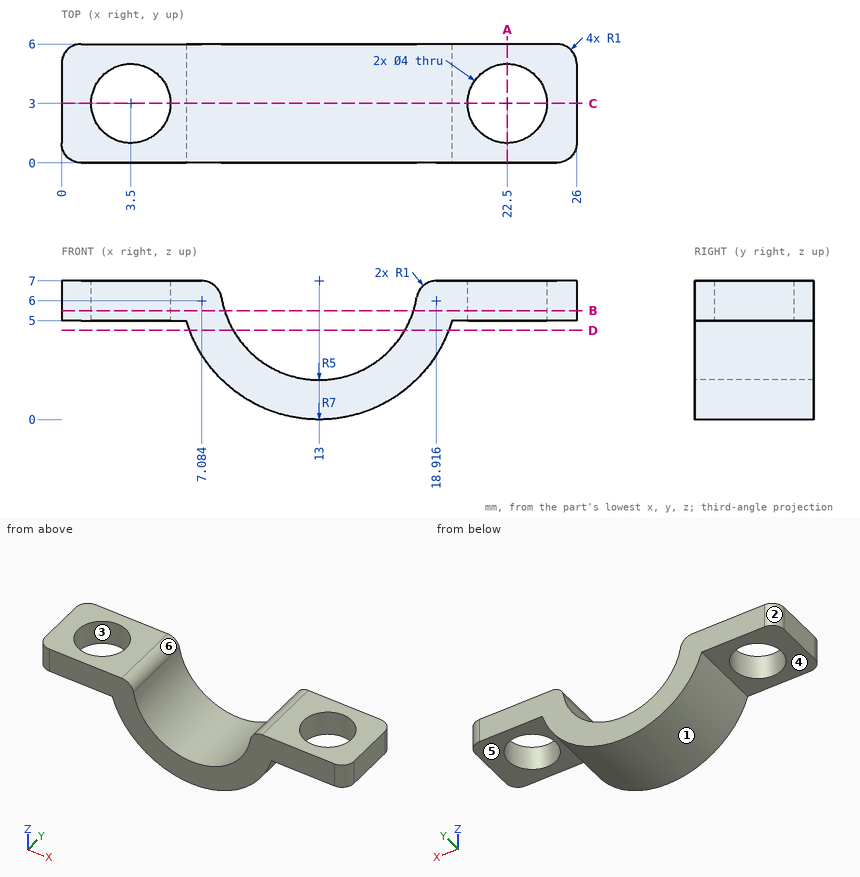
Drawing for the job (mm, zero at the part's lowest x, y, z). A direction names the side the tool comes from. Round coordinates to 2 decimals unless told otherwise and drop trailing zeros. Loops run counter-clockwise (first coordinate to the right, second up) from the corner with the lowest first, then second, coordinate; pieces in that order, holes last. Notation, with made-up numbers: (73, -38) -> (115, -38) arc R17 cw to (115, -19) -> close; hole circle Ø10 at (37, 24). An arc over 180 degrees is marked (long way). Use one line per item in the form item = value. Start each with the question number.
Item 1: Band-saw the part on D-D (z = 4.5). List the corners of the cut face in (x, y), plus the area to 3 significant figures.
Item 2: Band-saw the part on A-A (x = 22.5). List the corners of the cut face in (y, z), plus the area to 3 significant figures.
Item 3: Drop flat-ended pins along their axis: pin 1 Ø4 at (x, z) = (16, 4) entering from -Y; pin 2 Ø1.8 at (x, y) = (21.5, 1.5) entering from -Z; pin 3 Ø1 at (x, y) = (11, 4.5) entering from +Z; pin 4 Ø3.5 at (x, y) = (22.5, 3) entering from +Z. Give the stop position or say it passes through.
Item 4: Two-plate mould, pull along Y, no slides. Class the marked faces 1, 2 and 3: released by +Y, released by -Y, zero draft, split by the parting line, or undercut.
Item 5: Tool access for the marked faces 4, 5 and 6: list every direction of +Z, -Z, +X, -X, +Y, -Y with a clear straight run to the whole face (end or side of a thin tool).
Item 6: Band-saw the part on B-B (z = 5.5). List the corners of the cut face in (x, y).
Item 7: Band-saw the part on C-C (y = 3). List the corners of the cut face in (x, z).
Item 8: Drill centre lines: line 1 along Y through (x, z) = (22.5, 6.65); line 2 along X through (y, z) = (2.4, 6.75) (1 decimal); line 3 along X through (y, z) = (5.3, 5.5). Where is each one in solid material? Low to high.
Data:
q1.outline = (6.46, 0) -> (8.67, 0) -> (8.67, 6) -> (6.46, 6) -> close; (17.33, 0) -> (19.54, 0) -> (19.54, 6) -> (17.33, 6) -> close
q1.area = 26.5 mm^2
q2.outline = (0, 5) -> (1, 5) -> (1, 7) -> (0, 7) -> close; (5, 5) -> (6, 5) -> (6, 7) -> (5, 7) -> close
q2.area = 4.00 mm^2
q3.pin_1 = 0
q3.pin_2 = 5
q3.pin_3 = 2.67
q3.pin_4 = through
q4.face_1 = zero draft
q4.face_2 = released by +Y
q4.face_3 = undercut
q5.face_4 = -Z, -X, +Y, -Y
q5.face_5 = -Z, +X, +Y, -Y
q5.face_6 = +Z, +Y, -Y
q6.outline = (0, 1) arc R1 ccw to (1, 0) -> (8.23, 0) -> (8.23, 6) -> (1, 6) arc R1 ccw to (0, 5) -> close; (17.77, 0) -> (25, 0) arc R1 ccw to (26, 1) -> (26, 5) arc R1 ccw to (25, 6) -> (17.77, 6) -> close; hole circle Ø4 at (3.5, 3); hole circle Ø4 at (22.5, 3)
q7.outline = (0, 5) -> (1.5, 5) -> (1.5, 7) -> (0, 7) -> close; (5.5, 5) -> (6.29, 5) arc R7 ccw to (19.71, 5) -> (20.5, 5) -> (20.5, 7) -> (18.92, 7) arc R1 ccw to (17.93, 6.17) arc R5 cw to (8.07, 6.17) arc R1 ccw to (7.08, 7) -> (5.5, 7) -> close; (24.5, 5) -> (26, 5) -> (26, 7) -> (24.5, 7) -> close
q8.line_1 = 0 to 1, 5 to 6
q8.line_2 = 0 to 1.6, 5.4 to 7.7, 18.3 to 20.6, 24.4 to 26
q8.line_3 = 0.05 to 8.23, 17.77 to 25.95
